Model file for the job. Use its own axes, mm. Round coordinates to 2 decimals unless told otherwise and drop trailing zeros. Loops run counter-clockwise (first coordinate to the right, second up) from the corner with the lowest first, then second, coordinate; pieces in that order, holes last. Notation, with made-up numbers: (-4, -30) -> (46, -30) arc R22 ccw to (46, -20) -> close; hole circle Ø6 at (34.25, 81.5). An arc over 180 degrees is marked (long way). Use a Markdown table: item, result. Add a question column.
```python
from build123d import *

# Parameters (mm, degrees)
F0_W     = 57.5
F0_H     = 57.5
F0_R     = 2.5
F1_DEPTH = 5
F2_R     = 20
F3_DEPTH = 5


with BuildPart() as f1:
    # F0 (on Top) → F1 (new body)
    with BuildSketch(Plane.XY):
        with Locations((2.407941, 10.496731)):
            Rectangle(F0_W, F0_H)
        with Locations((-20.842059, -12.753269)):
            Circle(F0_R, mode=Mode.SUBTRACT)
        with Locations((26.157941, -12.753269)):
            Circle(F0_R, mode=Mode.SUBTRACT)
        with Locations((-20.842059, 34.246731)):
            Circle(F0_R, mode=Mode.SUBTRACT)
        with Locations((26.157941, 34.246731)):
            Circle(F0_R, mode=Mode.SUBTRACT)
    extrude(amount=F1_DEPTH)

    # F2 (on face) → F3 (cut)
    with BuildSketch(Plane.XY.offset(5)):
        with Locations((2.157941, 10.246731)):
            Circle(F2_R)
    extrude(amount=-F3_DEPTH, mode=Mode.SUBTRACT)

    # F4: F1 across face


with BuildPart() as f1_1:
    add(f1.part)
    add(f1.part.mirror(Plane(origin=(-26.342059, 10.496731, 2.5), x_dir=(0, -1, 0), z_dir=(-1, 0, 0))))


solid = f1_1.part
```
1) Cut at A-A on y = -6.5. Write the cut outline in (x, z), and give its area (3 significant figures).
2) Cut at B-B on x = -47.5. Write the cut outline in (y, z).
3) Cut at C-C on z = 3.9. Count the separate pieces of the cut face and the enclosed holes in it, and give its area (3 significant figures).
4) Pin check, flat tip, straight feed: pin 1 Ø4 at (x, y) = (-20.84, 34.25) entering from +Z. Stop position of the tip, or through.
5) Pull direction X, two halves, no side cores. Call faces 1 (the face through (24.32, -11.06, 2.46)), 2 (the face through (-26, 39.247, 2)), 3 (the face through (-83.842, 10, 2)): +X half, -X half, draft (parallel to the pull), parting line (faces both ways), or undercut.
6) Cut at D-D on y = 7.5. Write the cut outline in (x, z).
7) Wall check: probe 1 along X at (y, z) = (-12.5, 1); probe 2 along X at (y, z) = (9.5, 2.55); probe 3 along X at (y, z) = (1, 0.45). Give the ranges that are in metal, low to high. Write a range as from..to.
Established:
| question | item | result |
|---|---|---|
| 1 | outline | (-83.84, 0) -> (-65.78, 0) -> (-65.78, 5) -> (-83.84, 5) -> close; (-43.91, 0) -> (-8.78, 0) -> (-8.78, 5) -> (-43.91, 5) -> close; (13.09, 0) -> (31.16, 0) -> (31.16, 5) -> (13.09, 5) -> close |
| 1 | area | 356 mm^2 |
| 2 | outline | (-18.25, 0) -> (-8.36, 0) -> (-8.36, 5) -> (-18.25, 5) -> close; (28.85, 0) -> (39.25, 0) -> (39.25, 5) -> (28.85, 5) -> close |
| 3 | separate pieces | 1 |
| 3 | enclosed holes | 10 |
| 3 | area | 3,940 mm^2 |
| 4 | pin 1 | passes through |
| 5 | face 1 | undercut |
| 5 | face 2 | draft |
| 5 | face 3 | -X half |
| 6 | outline | (-83.84, 0) -> (-74.65, 0) -> (-74.65, 5) -> (-83.84, 5) -> close; (-35.03, 0) -> (-17.65, 0) -> (-17.65, 5) -> (-35.03, 5) -> close; (21.97, 0) -> (31.16, 0) -> (31.16, 5) -> (21.97, 5) -> close |
| 7 | probe 1 | x = -83.84..-81.33, -76.35..-34.33, -29.35..-23.33, -18.35..23.67, 28.65..31.16 |
| 7 | probe 2 | x = -83.84..-74.83, -34.86..-17.83, 22.14..31.16 |
| 7 | probe 3 | x = -83.84..-72.58, -37.11..-15.58, 19.89..31.16 |
